```python
from build123d import *

# Parameters (mm, degrees)
BOSS_EXTRUDE1_DEPTH = 189
SHELL2_T            = -0.3


with BuildPart() as part:
    # Sketch1 → Boss-Extrude1 (new body)
    with BuildSketch(Plane.XY):
        with BuildLine():
            Line((-50, -31.525272579), (50, -31.525272579))
            Line((50, -31.525272579), (50, 148.474727421))
            ThreePointArc((50, 148.474727421), (0, 198.474727421), (-50, 148.474727421))
            Line((-50, 148.474727421), (-50, -31.525272579))
        make_face()
    extrude(amount=BOSS_EXTRUDE1_DEPTH)

    # Shell2
    shell2_openings = [part.faces().sort_by_distance(p)[0] for p in [
        (0, 78.393671634, 189),
    ]]
    offset(amount=SHELL2_T, openings=shell2_openings, kind=Kind.INTERSECTION)


solid = part.part
```
Geometry: final body of the model. Coordinates: model frame, mm. A direction names the side the tool comes from. Coordinates: 2 decimals unless noted, no trailing zeros. Order: outer loops, then holes, each group sorted by start corner. A loop starts at its lowest first (then second) coordinate and runs counter-clockwise, first axis right, second up. Notation, with made-up numbers: M -36.5,52 L -27.5,52 A14 cw -27.5,76 Z; hole C 25.25,66.25 d1. An arc over 180 degrees is marked long. Answer in a Markdown table with one row per item. Add a question column.
Q1. Section query C-C on y = 134.5. Return the cut outline in (x, z), and give its area (3 significant figures).
Q2. Section query A-A on z = 154. Return the cut outline in (x, y), and give its area (3 significant figures).
Q3. Reachability of faces 1 (the flat face through (-1, 85, 0)), 2 (the cylindrical face through (1.093, 198.163, 93.329)) from +Z, -Z, +X, -X, +Y, -Y: full face, straight path, thin tool, end or side. Return the list, or none.
Q4. Line query: L1, parallel to X at y = 25, z = 47; L2, parallel to Y at x = 1, z = 39; L3, parallel to Y at x = 27, z = 106. Output: solid intervals per line, ascending.
Q5. Section query B-B on x = 0. Return the cut outline in (y, z).
Q6. Mould query, pull axis Y, two halves, no side actions, for faces 3 (the cylindrical face through (1.099, 198.463, 93.177)), 4 (the flat face through (-1, -31.525, 93)), 5 (the flat face through (-49.7, 60, 93)), 6 (the flat face through (50, 57, 93)). Classes: released by +Y, released by -Y, zero draft, split by the parting line, or undercut.
Q7. Contact query for a flat-ended pin moving along its axis: P1, Ø5, axis at x = 0.5, z = 97.5, coming from the +Y side. Output: stop coordinate, or through.
Completed:
| question | item | result |
|---|---|---|
| 1 | outline | M -50,0 L 50,0 L 50,189 L 49.7,189 L 49.7,0.3 L -49.7,0.3 L -49.7,189 L -50,189 Z |
| 1 | area | 143 mm2 |
| 2 | outline | M -50,-31.53 L 50,-31.53 L 50,148.47 A50 ccw -50,148.47 Z; hole M -49.7,-31.23 L 49.7,-31.23 L 49.7,148.47 A49.7 ccw -49.7,148.47 Z |
| 2 | area | 185 mm2 |
| 3 | face 1 | -Z, +X, -X, +Y, -Y |
| 3 | face 2 | +Z |
| 4 | L1 | x = -50 to -49.7, 49.7 to 50 |
| 4 | L2 | y = -31.53 to -31.23, 198.16 to 198.46 |
| 4 | L3 | y = -31.53 to -31.23, 190.2 to 190.56 |
| 5 | outline | M -31.53,0 L 198.47,0 L 198.47,189 L 198.17,189 L 198.17,0.3 L -31.23,0.3 L -31.23,189 L -31.53,189 Z |
| 6 | face 3 | released by +Y |
| 6 | face 4 | released by -Y |
| 6 | face 5 | undercut |
| 6 | face 6 | zero draft |
| 7 | P1 | stops at y = 198.47 |
